Geometry check sheet. Reference: the model listing, model coordinates, mm. A direction names the side the tool comes from. Coordinates: 2 decimals unless noted, no trailing zeros. Loops run counter-clockwise (first coordinate to the right, second up) from the corner with the lowest first, then second, coordinate; pieces in that order, holes last. Notation, with made-up numbers: M -22,-20.5 L -10,-20.5 A6 cw -10,-12.5 Z; hole C 9,15 d7. An arc over 180 degrees is marked long. Use CSV: the item, a comma, the result in double quotes.
```python
from build123d import *

# Parameters (mm, degrees)
SKETCH_1_W          = 9
SKETCH_1_H          = 9
EXTRUDE_1_DEPTH     = 16
SKETCH_2_W          = 7
SKETCH_2_H          = 7
CUT_EXTRUDE_1_DEPTH = 20
SKETCH_3_R          = 1.5
SKETCH_3_R_2        = 1.499605096
CUT_EXTRUDE_2_DEPTH = 20


with BuildPart() as part:
    # ｽｹｯﾁ1 → ﾎﾞｽ - 押し出し1 (new body)
    with BuildSketch(Plane.XY):
        Rectangle(SKETCH_1_W, SKETCH_1_H)
    extrude(amount=EXTRUDE_1_DEPTH)

    # ｽｹｯﾁ2 → ｶｯﾄ - 押し出し1 (cut)
    with BuildSketch(Plane.XY.offset(16)):
        Rectangle(SKETCH_2_W, SKETCH_2_H)
    extrude(amount=-CUT_EXTRUDE_1_DEPTH, mode=Mode.SUBTRACT)

    # ｽｹｯﾁ3 → ｶｯﾄ - 押し出し2 (cut)
    with BuildSketch(Plane(origin=(0, 4.5, 0), x_dir=(1, 0, 0), z_dir=(0, 1, 0))):
        with Locations((0, -3.5)):
            Circle(SKETCH_3_R)
        with Locations((0, -12.5)):
            Circle(SKETCH_3_R_2)
    extrude(amount=-CUT_EXTRUDE_2_DEPTH, mode=Mode.SUBTRACT)


solid = part.part
```
1. Gauge pin test, flat end, axial feed: P1, Ø3.5, axis at x = 0, z = 12.5, coming from the +Y side. Record the tip position at first contact, or that the pin passes through.
The answers:
P1,"y = 4.5"
2. Section check C-C, the plane z = 12.5. Record the cut outline in (x, y), plus the area to 3 significant figures.
The answers:
outline,"M -4.5,-4.5 L -1.5,-4.5 L -1.5,-3.5 L -3.5,-3.5 L -3.5,3.5 L -1.5,3.5 L -1.5,4.5 L -4.5,4.5 Z; M 1.5,-4.5 L 4.5,-4.5 L 4.5,4.5 L 1.5,4.5 L 1.5,3.5 L 3.5,3.5 L 3.5,-3.5 L 1.5,-3.5 Z"
area,"26.0 mm^2"
3. Set-up check for faces 1 (the flat face through (0, 3.5, 8)), 2 (the flat face through (4.5, 0, 8)): record each of +Z, -Z, +X, -X, +Y, -Y from which the full face is reachable in a straight line by a thin tool's end or side.
The answers:
face 1,"+Z, -Z"
face 2,"+Z, -Z, +X, +Y, -Y"
4. Release check for a two-part mould opening along Y. For faces 3 (the cylindrical face through (0, 4, 14)), 4 (the flat face through (-3.5, 0, 8)), 5 (the flat face through (0, 4.5, 8)) record: +Y half, -Y half, draft (parallel to the pull), parting line (faces both ways), or undercut.
The answers:
face 3,"draft"
face 4,"undercut"
face 5,"+Y half"
5. Thickness scan on line 1 (Z direction, x = 0, y = -3.7); line 2 (X direction, y = 3.95, z = 12.5); line 3 (Z direction, x = -0.5, y = -4). Record the ranges inside material, lowest first. Write a range as [from, to].
The answers:
line 1,"[0, 2], [5, 11], [14, 16]"
line 2,"[-4.5, -1.5], [1.5, 4.5]"
line 3,"[0, 2.09], [4.91, 11.09], [13.91, 16]"
6. Section check B-B, the plane x = 0. Record the cut outline in (y, z).
The answers:
outline,"M -4.5,0 L -3.5,0 L -3.5,2 L -4.5,2 Z; M -4.5,5 L -3.5,5 L -3.5,11 L -4.5,11 Z; M -4.5,14 L -3.5,14 L -3.5,16 L -4.5,16 Z; M 3.5,0 L 4.5,0 L 4.5,2 L 3.5,2 Z; M 3.5,5 L 4.5,5 L 4.5,11 L 3.5,11 Z; M 3.5,14 L 4.5,14 L 4.5,16 L 3.5,16 Z"
7. Section check A-A, the plane y = -3. Record the cut outline in (x, z), plus the area to 3 significant figures.
The answers:
outline,"M -4.5,0 L -3.5,0 L -3.5,16 L -4.5,16 Z; M 3.5,0 L 4.5,0 L 4.5,16 L 3.5,16 Z"
area,"32.0 mm^2"
